Autodesk Inventor part; units mm, degrees
ref_plane "YZ Plane" through (0, 0, 0) normal (1, 0, 0) x (0, 1, 0)
ref_plane "XZ Plane" through (0, 0, 0) normal (0, 1, 0) x (-1, 0, 0)
ref_plane "XY Plane" through (0, 0, 0) normal (0, 0, 1) x (1, 0, 0)
sketch "Sketch1" plane through (0, 0, 0) normal (0, 0, 1) x (1, 0, 0)
  line L0 (0, 0) -> (22.5, 0)
  line L1 (22.5, 0) -> (22.5, 22.5)
  line L2 (22.5, 22.5) -> (0, 22.5)
  line L3 (0, 22.5) -> (0, 0)
  line L4 (0, 0) -> (20.5, 0)
  line L5 (20.5, 0) -> (20.5, 2)
  line L6 (20.5, 2) -> (0, 2)
  line L7 (0, 2) -> (0, 0)
  line L8 (22.5, 0) -> (20.5, 0)
  line L9 (20.5, 0) -> (20.5, 20.5)
  line L10 (20.5, 20.5) -> (22.5, 20.5)
  line L11 (22.5, 20.5) -> (22.5, 0)
  line L12 (22.5, 22.5) -> (2, 22.5)
  line L13 (2, 22.5) -> (2, 20.5)
  line L14 (2, 20.5) -> (22.5, 20.5)
  line L15 (22.5, 20.5) -> (22.5, 22.5)
  line L16 (0, 22.5) -> (2, 22.5)
  line L17 (2, 22.5) -> (2, 2)
  line L18 (2, 2) -> (0, 2)
  line L19 (0, 2) -> (0, 22.5)
  line L20 (2, 2) -> (20.5, 2)
  line L21 (20.5, 2) -> (20.5, 20.5)
  line L22 (20.5, 20.5) -> (2, 20.5)
  line L23 (2, 20.5) -> (2, 2)
  dimension "d0" = 22.5
  dimension "d1" = 22.5
  dimension "d2" = 20.5
  dimension "d3" = 2
  dimension "d4" = 2
  dimension "d5" = 20.5
  dimension "d6" = 20.5
  dimension "d7" = 2
  dimension "d8" = 2
  dimension "d9" = 20.5
  dimension "d10" = 18.5
  dimension "d11" = 18.5
extrude "Extrusion1" add sketch "Sketch1" along normal blind 86.75
sketch "Sketch6" plane through (0, 0, 0) normal (0, -1, 0) x (1, 0, 0)
  line L0 (0, 0) -> (22.5, 0)
  line L1 (0, 0) -> (20.5, 0)
  line L2 (20.5, 0) -> (20.5, 2)
  line L3 (20.5, 2) -> (0, 2)
  line L4 (0, 2) -> (0, 0)
  line L5 (22.5, 0) -> (22.5, 86.75)
  line L6 (22.5, 0) -> (20.5, 0)
  line L7 (20.5, 0) -> (20.5, 84.75)
  line L8 (20.5, 84.75) -> (22.5, 84.75)
  line L9 (22.5, 84.75) -> (22.5, 0)
  line L10 (22.5, 86.75) -> (2, 86.75)
  line L11 (2, 86.75) -> (2, 84.75)
  line L12 (2, 84.75) -> (22.5, 84.75)
  line L13 (22.5, 84.75) -> (22.5, 86.75)
  line L14 (0, 0) -> (0, 86.75)
  line L15 (0, 86.75) -> (2, 86.75)
  line L16 (2, 86.75) -> (2, 2)
  line L17 (2, 2) -> (0, 2)
  line L18 (0, 2) -> (0, 86.75)
  line L19 (20.5, 84.75) -> (2, 84.75)
  line L20 (2, 84.75) -> (2, 2)
  line L21 (2, 2) -> (20.5, 2)
  line L22 (20.5, 2) -> (20.5, 84.75)
  dimension "d28" = 20.5
  dimension "d29" = 2
  dimension "d30" = 2
  dimension "d31" = 84.75
  dimension "d32" = 20.5
  dimension "d33" = 2
  dimension "d34" = 2
  dimension "d35" = 84.75
  dimension "d36" = 18.5
  dimension "d37" = 82.75
extrude "Extrusion5" cut sketch "Sketch6" against normal blind 20.5 contours L3 L16 L12 L7
chamfer "Chamfer1" distance 1.5 angle 45 4 edges at (11.25, 22.5, 0) (22.5, 22.5, 43.375) (0, 22.5, 43.375) (11.25, 22.5, 86.75)
chamfer "Chamfer2" distance 1 angle 45 4 edges at (0, 10.5, 86.75) (22.5, 10.5, 86.75) (0, 10.5, 0) (22.5, 10.5, 0)
chamfer "Chamfer3" distance 0.8165 angle 45 4 edges at (1, 22, 85.75) (21.5, 22, 85.75) (21.5, 22, 1) (1, 22, 1)
properties part number "1-Battery-Case"
Geometry check sheet. Reference: the model listing, model coordinates, mm. A direction names the side the tool comes from. Round coordinates to 2 decimals unless told otherwise and drop trailing zeros. Order: outer loops, then holes, each group sorted by start corner. A loop starts at its lowest first (then second) coordinate and runs counter-clockwise, first axis right, second up. Notation, with made-up numbers: (40, 20) - (95, 20) arc R34 cw to (95, 58) - close; hole circle Ø10 at (9.25, 52). An arc over 180 degrees is marked (long way). Use a Markdown table: item, result. Add a question column.
(1) Sectioned sample at B-B, the plane z = 54. Enter the section's corners in (x, y), and give its area (3 significant figures).
(2) Tool access check on faces 1 (the flat face through (11, 10, 2)), 2 (the flat face through (22.5, 10, 43)). Record the directions out of +Z, -Z, +X, -X, +Y, -Y that give a thin tool (end or side, any length) a straight path to the whole face; none if there is none.
(3) Material ranges on line 1 along Z through (x, y) = (8.75, 9); line 2 along X through (y, z) = (6.25, 61); line 3 along Y through (x, z) = (19.5, 23.5), recorded low to high. Write a range as [from, to].
(4) Release check for a two-part mould opening along X. For faces 3 (the flat face through (11, 20.5, 44)), 4 (the flat face through (21.8, 21.7, 42.8)), 5 (the flat face through (11, 22.5, 43)) record: pulls with the +X half, pulls with the -X half, needs draft (parallel to the pull), parting line crosses it, or undercut.
(5) Sectioned sample at C-C, the plane x = 6.75. Enter the section's corners in (y, z), and give its area (3 significant figures).
(6) Sectioned sample at A-A, the plane y = 7. Enter the section's corners in (x, z), and give its area (3 significant figures).
(7) Depth check by flat-ended pin: pin 1 (8 mm diameter, centred on x = 11.5, z = 17.5, fed in from -Y); pin 2 (1.5 mm diameter, centred on x = 16.5, y = 12, fed in from -Z). Enter the tip coordinate at first touch or a pass-through.
Answers below:
| question | item | result |
|---|---|---|
| 1 | outline | (0, 0) - (2, 0) - (2, 20.5) - (20.5, 20.5) - (20.5, 0) - (22.5, 0) - (22.5, 21) - (21, 22.5) - (1.5, 22.5) - (0, 21) - close |
| 1 | area | 125 mm² |
| 2 | face 1 | -Y |
| 2 | face 2 | +Z, -Z, +X, +Y, -Y |
| 3 | line 1 | [0, 2], [84.75, 86.75] |
| 3 | line 2 | [0, 2], [20.5, 22.5] |
| 3 | line 3 | [20.5, 22.5] |
| 4 | face 3 | undercut |
| 4 | face 4 | pulls with the +X half |
| 4 | face 5 | needs draft |
| 5 | outline | (0, 0) - (21, 0) - (22.5, 1.5) - (22.5, 85.25) - (21, 86.75) - (0, 86.75) - (0, 84.75) - (20.5, 84.75) - (20.5, 2) - (0, 2) - close |
| 5 | area | 253 mm² |
| 6 | outline | (0, 1) - (1, 0) - (21.5, 0) - (22.5, 1) - (22.5, 85.75) - (21.5, 86.75) - (1, 86.75) - (0, 85.75) - close; hole (2, 2) - (20.5, 2) - (20.5, 84.75) - (2, 84.75) - close |
| 6 | area | 419 mm² |
| 7 | pin 1 | y = 20.5 |
| 7 | pin 2 | z = 0 |
